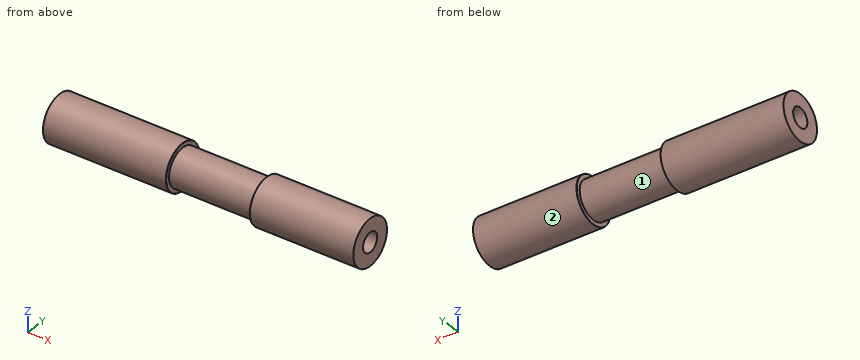
```python
from build123d import *

# Parameters (mm, degrees)
F0_R     = 5.925
F1_DEPTH = 31.678
F2_R     = 4.865
F3_DEPTH = 21.553
F4_R     = 5.95
F4_R_2   = 4.865
F5_DEPTH = 26.679
F7_D     = 5
F8_SIZE  = 0.05
F9_SIZE  = 0.05


with BuildPart() as f1:
    # F0 (on Right) → F1 (new body)
    with BuildSketch(Plane.YZ):
        Circle(F0_R)
    extrude(amount=F1_DEPTH)

    # F2 (on face) → F3 (join)
    with BuildSketch(Plane.YZ.offset(31.678)):
        Circle(F2_R)
    extrude(amount=F3_DEPTH)

    # F4 (on face) → F5 (join)
    with BuildSketch(Plane.YZ.offset(53.231)):
        Circle(F4_R)
        Circle(F4_R_2, mode=Mode.SUBTRACT)
        Circle(F4_R_2)
    extrude(amount=F5_DEPTH)

    # F7 (through all)
    with Locations(Plane.YZ.offset(79.91)):
        with Locations((0, 0)):
            Hole(F7_D / 2)

    # F8
    f8_edges = [f1.edges().sort_by_distance(p)[0] for p in [
        (31.678, -5.925, 0),
    ]]
    chamfer(f8_edges, length=F8_SIZE)

    # F9
    f9_edges = [f1.edges().sort_by_distance(p)[0] for p in [
        (53.231, -5.95, 0),
    ]]
    chamfer(f9_edges, length=F9_SIZE)


solid = f1.part
```
Geometry check sheet. Reference: the model listing, model coordinates, mm. Face numbers are marked on the shaded views. A direction names the side the tool comes from. Round coordinates to 2 decimals unless told otherwise and drop trailing zeros. Order: outer loops, then holes, each group sorted by start corner. A loop starts at its lowest first (then second) coordinate and runs counter-clockwise, first axis right, second up. Notation, with made-up numbers: (-3.5, 41) -> (44.5, 41) arc R7 ccw to (44.5, 45) -> close; hole circle Ø7 at (-10.75, 17.5). An arc over 180 degrees is marked (long way). Return JSON: item names as keys, results as strings. Group by question number.
Q1. Gauge pin test, flat ends, axial feed: pin 1 (4 mm diameter, centred on y = 3, z = -3.5, fed in from -X); pin 2 (1.5 mm diameter, centred on x = 26, z = -1, fed in from -Y); pin 3 (4 mm diameter, centred on y = 0, z = 0, fed in from -X); pin 4 (5 mm diameter, centred on x = 41.5, z = -2.5, fed in from -Y) (3 decimals). Record the tip position at first contact, or that the pin passes through.
Q2. Section check D-D, the plane x = 65. Record the boundary of the cut face in (y, z), plus the area to 3 significant figures.
Q3. Tool access check on the marked faces 1 and 2. Record the directions out of +Z, -Z, +X, -X, +Y, -Y that give a thin tool (end or side, any length) a straight path to the whole face; none if there is none.
Q4. Section check C-C, the plane x = 13. Record the boundary of the cut face in (y, z) (3 decimals).
Q5. Section check A-A, the plane z = 0. Record the boundary of the cut face in (x, y) (3 decimals), plus the area to 3 significant figures.
Q6. Material ranges on probe 1 along X at (y, z) = (-3, -4.5); probe 2 along Z at (x, y) = (55, 0); probe 3 along Z at (x, y) = (40.5, 0) (3 decimals), recorded low to high. Write a range as from..to.
Numbers:
{
 "1": {"pin 1": "x = 0", "pin 2": "y = -5.92", "pin 3": "through", "pin 4": "y = -4.865"},
 "2": {"outline": "circle Ø11.9 at (0, 0); hole circle Ø5 at (0, 0)", "area": "91.6 mm^2"},
 "3": {"face 1": "none", "face 2": "+X, -X"},
 "4": {"outline": "circle Ø11.85 at (0, 0); hole circle Ø5 at (0, 0)"},
 "5": {"outline": "(0, -5.925) -> (31.628, -5.925) -> (31.678, -5.875) -> (31.678, -4.865) -> (53.231, -4.865) -> (53.231, -5.9) -> (53.281, -5.95) -> (79.91, -5.95) -> (79.91, -2.5) -> (0, -2.5) -> close; (0, 2.5) -> (79.91, 2.5) -> (79.91, 5.95) -> (53.281, 5.95) -> (53.231, 5.9) -> (53.231, 4.865) -> (31.678, 4.865) -> (31.678, 5.875) -> (31.628, 5.925) -> (0, 5.925) -> close", "area": "503 mm^2"},
 "6": {"probe 1": "0..31.68, 53.23..79.91", "probe 2": "-5.95..-2.5, 2.5..5.95", "probe 3": "-4.865..-2.5, 2.5..4.865"}
}
